Answer from the drawing. Dimensions are ordinates in mm from the lowest x, y and z of the part. A direction names the side the tool comes from. Coordinates: 2 decimals unless noted, no trailing zeros. Loops run counter-clockwise (first coordinate to the right, second up) from the corner with the lowest first, then second, coordinate; pieces in that order, holes last.
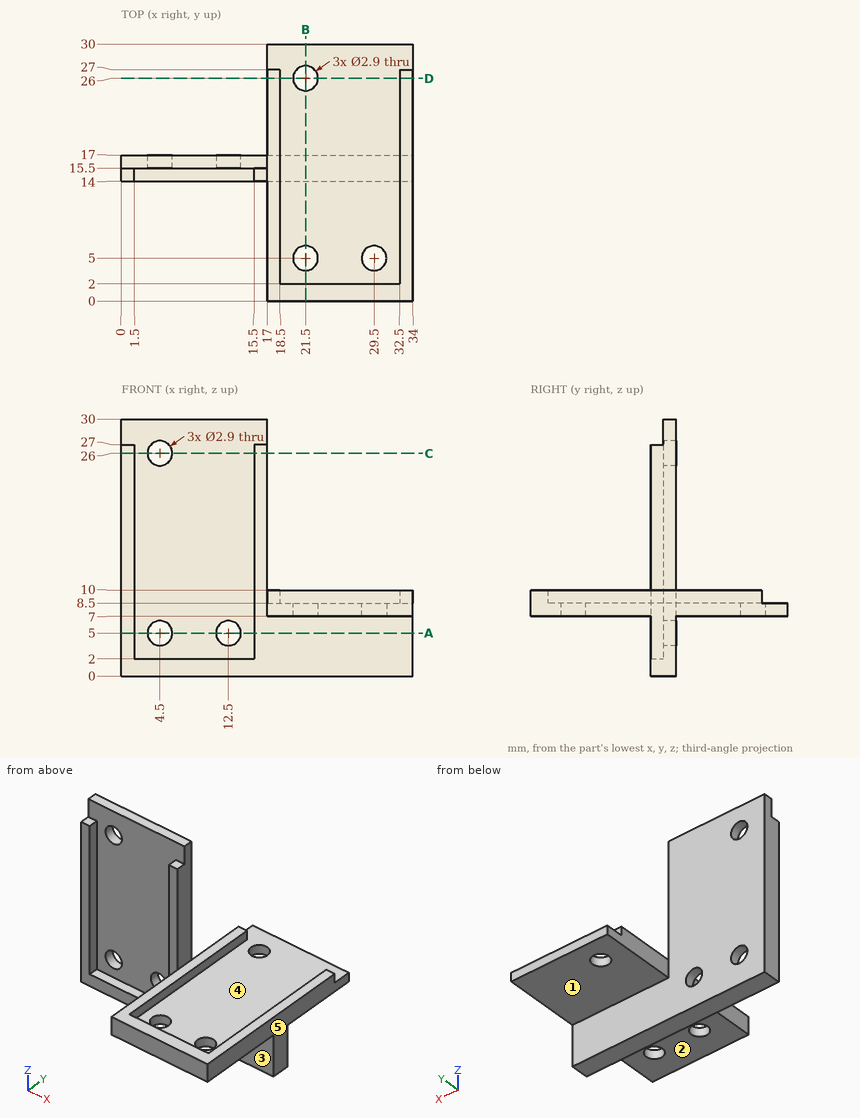
Item 1: A cutting plane is placed at C-C on z = 26. Determine the outline of the cut face in (x, y).
Numbers:
outline: (0, 14) - (1.5, 14) - (1.5, 15.5) - (3.05, 15.5) - (3.05, 17) - (0, 17) - close; (5.95, 15.5) - (15.5, 15.5) - (15.5, 14) - (17, 14) - (17, 17) - (5.95, 17) - close
Item 2: Find the intervals of material crossed by line 1 along Y through (x, z) = (21.5, 7.55); line 2 along X through (y, z) = (21, 9), in increasing order.
Numbers:
line 1: y = 0 to 3.55, 6.45 to 24.55, 27.45 to 30
line 2: x = 17 to 18.5, 32.5 to 34
Item 3: Given pin 1 (0.8 mm diameter, centred on x = 24, z = 9, fed in from +Y); pin 2 (10 mm diameter, centred on x = 25, y = 27, fed in from +Z); pin 3 (1.5 mm diameter, centred on x = 27.5, y = 26, fed in from -Z), each flat-ended and moving along its own axis, determine where each tip first touches the part or whether it passes through.
Numbers:
pin 1: stops at y = 2
pin 2: stops at z = 8.5
pin 3: stops at z = 7
Item 4: A cutting plane is placed at B-B on x = 21.5. Determine the outline of the cut face in (y, z), then the cut area to 3 significant figures.
Numbers:
outline: (0, 7) - (3.55, 7) - (3.55, 8.5) - (2, 8.5) - (2, 10) - (0, 10) - close; (6.45, 7) - (14, 7) - (14, 0) - (17, 0) - (17, 7) - (24.55, 7) - (24.55, 8.5) - (6.45, 8.5) - close; (27.45, 7) - (30, 7) - (30, 8.5) - (27.45, 8.5) - close
area: 60.3 mm2
Item 5: Which of the six approach directions +Z, -Z, +X, -X, +Y, -Y give full straight-line access (tool end or side, diameter ignored) to the marked faces 1 and 2?
Numbers:
face 1: -Z, +X, -X, +Y
face 2: -Z, +X, -X, -Y
Item 6: A cutting plane is placed at A-A on z = 5. Determine the outline of the cut face in (x, y), then the cut area to 3 significant figures.
Numbers:
outline: (0, 14) - (1.5, 14) - (1.5, 15.5) - (3.05, 15.5) - (3.05, 17) - (0, 17) - close; (5.95, 15.5) - (11.05, 15.5) - (11.05, 17) - (5.95, 17) - close; (13.95, 15.5) - (15.5, 15.5) - (15.5, 14) - (34, 14) - (34, 17) - (13.95, 17) - close
area: 72.3 mm2
Item 7: Determine the mould class of the marked faces 3, 4 and 5 for opening direction X: released by +X, released by -X, zero draft, split by the parting line, or undercut.
Numbers:
face 3: zero draft
face 4: undercut
face 5: released by +X
Item 8: A cutting plane is placed at D-D on y = 26. Determine the outline of the cut face in (x, z).
Numbers:
outline: (17, 7) - (20.05, 7) - (20.05, 8.5) - (18.5, 8.5) - (18.5, 10) - (17, 10) - close; (22.95, 7) - (34, 7) - (34, 10) - (32.5, 10) - (32.5, 8.5) - (22.95, 8.5) - close
